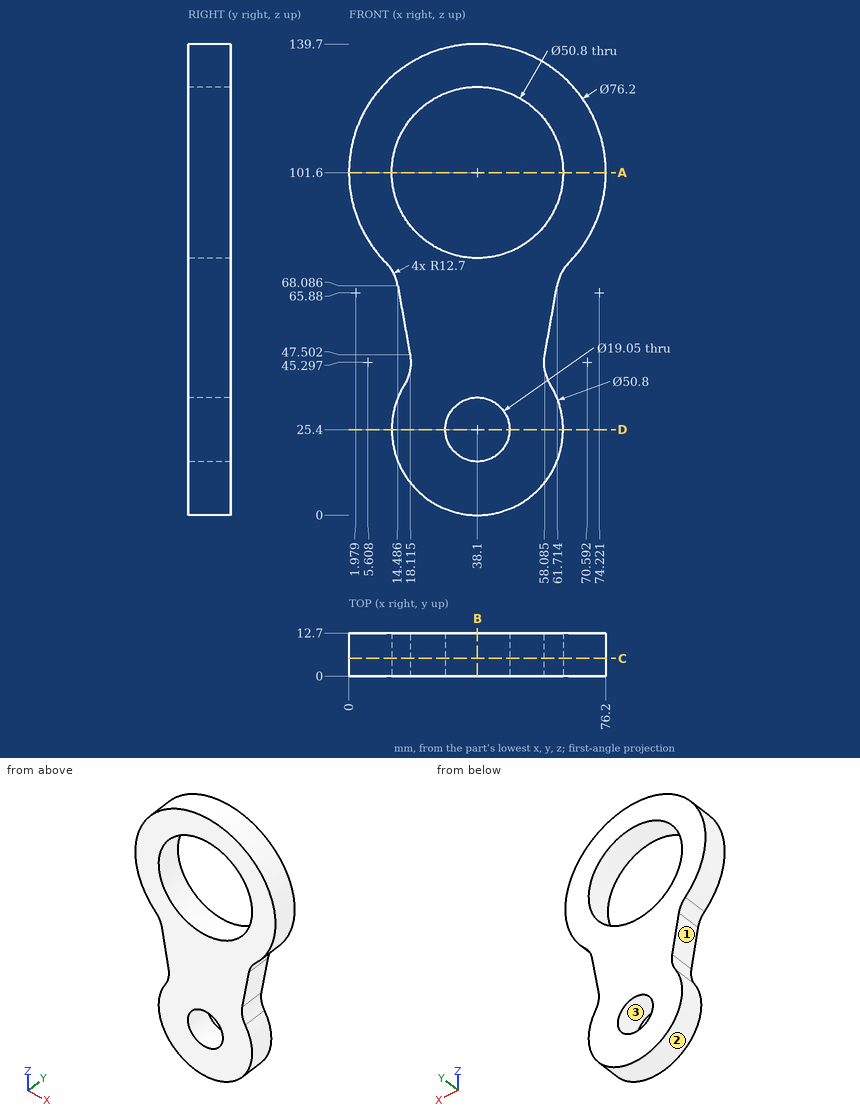
Here's the drawing with two shaded views (mm, measured from the low corner). I have some questions. Round coordinates to 2 decimals unless told otherwise and drop trailing zeros. Loops run counter-clockwise (first coordinate to the right, second up) from the corner with the lowest first, then second, coordinate; pieces in that order, holes last.
Item 1: Will these pins go through, and if not, where does the flat tip stop? pin 1 Ø5 at (x, y) = (8, 3.5) entering from +Z (1 decimal); pin 2 Ø2 at (y, z) = (2.5, 76.5) entering from +X; pin 3 Ø4 at (x, y) = (27, 10.5) entering from +Z.
Item 2: Please list where these lines run through material, in increasing order: L1, parallel to X at y = 7, z = 25.4 (1 decimal); L2, parallel to X at y = 4.75, z = 101.6; L3, parallel to Z at x = 44.5, y = 6 (1 decimal).
Item 3: Suppose I cut it at D-D, the plane z = 25.4. Write out the boundary of the cut face in (x, y) (1 decimal), then the cut area to 3 significant figures.
Item 4: If we mould it in two halves opening along X, with no side actions, what happens to the marked faces 1, 2 and 3? For each: +X half, -X half, draft (parallel to the pull), parting line (faces both ways), or undercut.
Item 5: Suppose I cut it at B-B, the plane x = 38.1. Write out the boundary of the cut face in (y, z) (1 decimal), then the cut area to 3 significant figures.
Item 6: Suppose I cut it at C-C, the plane y = 5.25. State how many separate pieces and enclosed holes the cut face has, then the cut area to 3 significant figures.
Item 7: Suppose I cut it at A-A, the plane z = 101.6. Write out the boundary of the cut face in (x, y).
Reported:
1. pin 1: stops at z = 127.9
1. pin 2: stops at x = 67.61
1. pin 3: stops at z = 138.6
2. L1: x = 12.7 to 28.6, 47.6 to 63.5
2. L2: x = 0 to 12.7, 63.5 to 76.2
2. L3: z = 0.8 to 18.3, 32.5 to 77, 126.2 to 139.2
3. outline: (12.7, 0) - (28.6, 0) - (28.6, 12.7) - (12.7, 12.7) - close; (47.6, 0) - (63.5, 0) - (63.5, 12.7) - (47.6, 12.7) - close
3. area: 403 mm2
4. face 1: -X half
4. face 2: parting line
4. face 3: undercut
5. outline: (0, 0) - (12.7, 0) - (12.7, 15.9) - (0, 15.9) - close; (0, 34.9) - (12.7, 34.9) - (12.7, 76.2) - (0, 76.2) - close; (0, 127) - (12.7, 127) - (12.7, 139.7) - (0, 139.7) - close
5. area: 887 mm2
6. separate pieces: 1
6. enclosed holes: 2
6. area: 5,070 mm2
7. outline: (0, 0) - (12.7, 0) - (12.7, 12.7) - (0, 12.7) - close; (63.5, 0) - (76.2, 0) - (76.2, 12.7) - (63.5, 12.7) - close
